Design review of the part built by this model. Coordinates are the model's own, in mm. A direction names the side the tool comes from. Coordinates: 2 decimals unless noted, no trailing zeros. Order: outer loops, then holes, each group sorted by start corner. A loop starts at its lowest first (then second) coordinate and runs counter-clockwise, first axis right, second up. Notation, with made-up numbers: M 66,-5.75 L 100,-5.75 A27 ccw 100,10.25 Z; hole C 39.5,-13.5 d6. An arc over 180 degrees is marked long. Use CSV: the item, a comma, the result in double quotes.
```python
from build123d import *

# Parameters (mm, degrees)
SKETCH_2_W          = 9.723167254
SKETCH_2_H          = 12
EXTRUDE_1_DEPTH     = 2
SKETCH_3_R          = 4
EXTRUDE_2_DEPTH     = 4
SKETCH_4_R          = 2
EXTRUDE_3_DEPTH     = 7.4
FILLET_1_R          = 0.4
SKETCH_5_R          = 1.1
CUT_EXTRUDE_1_DEPTH = 2


with BuildPart() as part:
    # Эскиз2 → Бобышка-Вытянуть1 (new body)
    with BuildSketch(Plane.XY):
        Rectangle(SKETCH_2_W, SKETCH_2_H)
    extrude(amount=EXTRUDE_1_DEPTH)

    # Эскиз3 → Бобышка-Вытянуть2 (add)
    with BuildSketch(Plane.XY.offset(2)):
        with Locations((-0.238416373, -0.5)):
            Circle(SKETCH_3_R)
        Polygon((-3.084826535, -2.230127019), (-0.238416373, 2.7), (2.607993788, -2.230127019), align=None, mode=Mode.SUBTRACT)
    extrude(amount=EXTRUDE_2_DEPTH)

    # Эскиз4 → Бобышка-Вытянуть3 (add)
    with BuildSketch(Plane(origin=(0, 0, 0), x_dir=(-1, 0, 0), z_dir=(0, 0, -1))):
        with Locations(Location((-2.861583627, -0.5, 0), (0, 0, 180))):
            Circle(SKETCH_4_R)
    extrude(amount=EXTRUDE_3_DEPTH)

    # Скругление1
    fillet_1_edges = [part.edges().sort_by_distance(p)[0] for p in [
        (-4.238416373, -0.5, 6),
    ]]
    fillet(fillet_1_edges, radius=FILLET_1_R)

    # Эскиз5 → Вырез-Вытянуть1 (cut)
    with BuildSketch(Plane.XY.offset(2)):
        with Locations((-0.238416373, -0.58)):
            Circle(SKETCH_5_R)
    extrude(amount=-CUT_EXTRUDE_1_DEPTH, mode=Mode.SUBTRACT)


solid = part.part
```
(1) Add section C-C on x = 4.25. State the section outline as (y, z) points, and give its area (3 significant figures).
The answers:
outline,"M -6,0 L -1.94,0 L -1.94,-7.4 L 0.94,-7.4 L 0.94,0 L 6,0 L 6,2 L -6,2 Z"
area,"45.3 mm2"
(2) Clearance check with flat-ended pins moving along their axes: P1, Ø2, axis at x = 2.5, z = -1.5, coming from the +Y side; P2, Ø3, axis at x = -1, y = 0.5, coming from the -Z side; P3, Ø4, axis at y = 4, z = -5.5, coming from the -X side; P4, Ø1.2, axis at x = 0.5, z = 4, coming from the +Y side. State where each tip first meets the part, or that it passes through.
The answers:
P1,"stops at y = 1.5"
P2,"stops at z = 0"
P3,"passes through"
P4,"stops at y = 3.5"
(3) Wall thickness on probe 1 along Z at (x, y) = (4.75, -1); probe 2 along Y at (x, z) = (3, -0.5); probe 3 along Z at (x, y) = (-3, -1): over which ranges is each line inside the solid? List them lowest first.
The answers:
probe 1,"z = -7.4 to 2"
probe 2,"y = -2.5 to 1.5"
probe 3,"z = 0 to 6"
(4) Add section D-D on z = -4.5. State the section outline as (x, y) points.
The answers:
outline,"C 2.86,-0.5 d4"
(5) The part is to be moulded in two halves that separate along Y. For faces 1 (the face through (4.862, 0, 1)), 2 (the face through (-1.337, -0.532, 1.014)), 3 (the face through (-1.106, -4.405, 3.775)), 4 (the face through (0, -2.23, 4)), say which applies: pulls with the +Y half, pulls with the -Y half, needs draft (parallel to the pull), parting line crosses it, or undercut.
The answers:
face 1,"needs draft"
face 2,"undercut"
face 3,"parting line crosses it"
face 4,"undercut"
(6) For faces 5 (the face through (3, -1, -7.4)), 6 (the face through (0.864, -0.588, -3.648)), 7 (the face through (1.165, 0.269, 3.972)), list the 3-axis set-ups (+Z, -Z, +X, -X, +Y, -Y) from which the entire face can be reached by the end or side of a thin tool; tool diameter is ignored.
The answers:
face 5,"-Z, +X, -X, +Y, -Y"
face 6,"-Z"
face 7,"+Z"
(7) Add section A-A on y = -5. State the section outline as (x, z) points.
The answers:
outline,"M -4.86,0 L 4.86,0 L 4.86,2 L -4.86,2 Z"
(8) Add section B-B on z = 5.25. State the section outline as (x, y) points, and give its area (3 significant figures).
The answers:
outline,"C -0.24,-0.5 d8; hole M -3.08,-2.23 L 2.61,-2.23 L -0.24,2.7 Z"
area,"36.2 mm2"
